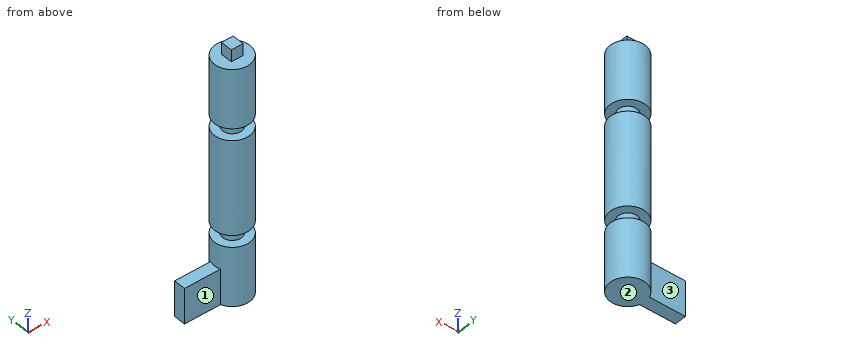
```python
from build123d import *

# Parameters (mm, degrees)
F0_R      = 7.5
F1_DEPTH  = 20
F2_R      = 4
F3_DEPTH  = 5
F4_R      = 7.5
F4_R_2    = 4
F5_DEPTH  = 25
F7_W      = 5
F7_H      = 5
F8_DEPTH  = 5
F9_W      = 24.7944914738
F9_H      = 5
F10_DEPTH = 15


with BuildPart() as f1:
    # F0 (on Top) → F1 (new body)
    with BuildSketch(Plane.XY):
        Circle(F0_R)
    extrude(amount=F1_DEPTH)

    # F2 (on face) → F3 (join)
    with BuildSketch(Plane.XY.offset(20)):
        Circle(F2_R)
    extrude(amount=F3_DEPTH)

    # F4 (on face) → F5 (join)
    with BuildSketch(Plane.XY.offset(25)):
        Circle(F4_R)
        Circle(F4_R_2, mode=Mode.SUBTRACT)
        Circle(F4_R_2)
    extrude(amount=F5_DEPTH)

    # F6: F1 across plane


with BuildPart() as f1_1:
    add(f1.part)
    add(f1.part.mirror(Plane.XY))

    # F7 (on face) → F8 (join)
    with BuildSketch(Plane.XY.offset(50)):
        Rectangle(F7_W, F7_H)
    extrude(amount=F8_DEPTH)

    # F9 (on face) → F10 (join)
    with BuildSketch(Plane(origin=(0, 0, -50), x_dir=(1, 0, 0), z_dir=(0, 0, -1))):
        with Locations((-9.8972457369, 0)):
            Rectangle(F9_W, F9_H)
    extrude(amount=-F10_DEPTH)


solid = f1_1.part
```
The listing builds one solid part. Answer for the finished solid, in the listing's coordinates (mm). Face numbers are marked on the shaded views. A direction names the side the tool comes from. Give positions to 0.01 mm unless a question says otherwise; leave off trailing zeros. Loops run counter-clockwise (first coordinate to the right, second up) from the corner with the lowest first, then second, coordinate; pieces in that order, holes last. Notation, with made-up numbers: M 44,78 L 57,78 A26 ccw 57,114 Z; hole C 25.5,71 d3. An arc over 180 degrees is marked long. One line per item, written item: value.
1. Section A-A on y = 5.25 is taken. Determine the outline of the cut face in (x, z).
Found:
outline: M -5.36,-50 L 5.36,-50 L 5.36,-25 L -5.36,-25 Z; M -5.36,-20 L 5.36,-20 L 5.36,20 L -5.36,20 Z; M -5.36,25 L 5.36,25 L 5.36,50 L -5.36,50 Z
2. For the marked faces 1, 2 and 3, determine the directions among +Z, -Z, +X, -X, +Y, -Y from which every point of the face is accessible in a straight line to the end or side of a thin tool.
Found:
face 1: +Z, -Z, -X, -Y
face 2: -Z, +X, -X, +Y, -Y
face 3: +Z, -Z, -X, +Y
3. Each of these flat-tipped pins is pushed along its axis until it touches: P1, Ø8, axis at x = -9, y = -3, coming from the +Z side; P2, Ø1, axis at y = -2, z = 25, coming from the +X side; P3, Ø3, axis at y = -4.5, z = -7.5, coming from the -X side. Where does it stop, or does it pass through?
Found:
P1: z = 50
P2: x = 7.35
P3: x = -6.87
4. Section B-B on x = 0 is taken. Determine the outline of the cut face in (y, z), plus the area to 4 significant figures.
Found:
outline: M -7.5,-50 L 7.5,-50 L 7.5,-25 L 4,-25 L 4,-20 L 7.5,-20 L 7.5,20 L 4,20 L 4,25 L 7.5,25 L 7.5,50 L 2.5,50 L 2.5,55 L -2.5,55 L -2.5,50 L -7.5,50 L -7.5,25 L -4,25 L -4,20 L -7.5,20 L -7.5,-20 L -4,-20 L -4,-25 L -7.5,-25 Z
area: 1,455 mm^2
5. Section D-D on z = 24 is taken. Determine the outline of the cut face in (x, y).
Found:
outline: C 0,0 d8
6. Section C-C on y = 0 is taken. Determine the outline of the cut face in (x, z), plus the area to 3 significant figures.
Found:
outline: M -22.29,-50 L 7.5,-50 L 7.5,-25 L 4,-25 L 4,-20 L 7.5,-20 L 7.5,20 L 4,20 L 4,25 L 7.5,25 L 7.5,50 L 2.5,50 L 2.5,55 L -2.5,55 L -2.5,50 L -7.5,50 L -7.5,25 L -4,25 L -4,20 L -7.5,20 L -7.5,-20 L -4,-20 L -4,-25 L -7.5,-25 L -7.5,-35 L -22.29,-35 Z
area: 1,680 mm^2
7. Find the intervals of material crossed by probe 1 along Z at (x, y) = (-5, 4.25); probe 2 along Y at (x, z) = (-16.5, -36.5); probe 3 along Y at (x, z) = (2.5, -28), in increasing order.
Found:
probe 1: -50 to -25, -20 to 20, 25 to 50
probe 2: -2.5 to 2.5
probe 3: -7.07 to 7.07
